Print and shaded views of the part. All mm, measured from the part's lowest x, y and z. A direction names the side the tool comes from. Coordinates: 2 decimals unless noted, no trailing zeros. Loops run counter-clockwise (first coordinate to the right, second up) from the corner with the lowest first, then second, coordinate; pieces in that order, holes last.
1) Saw through at C-C, the plane z = 6. Write the cut outline in (x, y), and give its area (3 significant figures).
2) Two-plate mould, pull along X, no slides. Class the marked faces 6, 7 and 8: +X half, -X half, draft (parallel to the pull), parting line (faces both ways), or undercut.
3) Saw through at D-D, the plane z = 10. Write the cut outline in (x, y), and give its area (3 significant figures).
4) Pin check, flat tips, straight feed: pin 1 Ø2 at (x, z) = (66, 2) entering from +Y; pin 2 Ø2.5 at (x, z) = (6, 6) entering from -Y; pin 3 Ø6 at (y, z) = (9, 5.5) entering from +X; pin 4 Ø6 at (y, z) = (9, 7) entering from -X. Stop position of each tip, or through.
5) Saw through at A-A, the plane y = 1.5. Write the cut outline in (x, z), and give its area (3 significant figures).
6) Which spindle directions (+Z, -Z, +X, -X, +Y, -Y) get a long thin tool onto all of the face, cutting with end or side? Do the marked faces 1, 2, 3, 4 and 5. Say none if no direction does.
7) Wall check: line 1 along Z through (x, y) = (6, 1.6); line 2 along X through (y, z) = (9.25, 7.75); line 3 along X through (y, z) = (10.75, 11). Give the ranges that are in metal, low to high.
8) Saw through at B-B, the plane x = 68. Write the cut outline in (y, z).
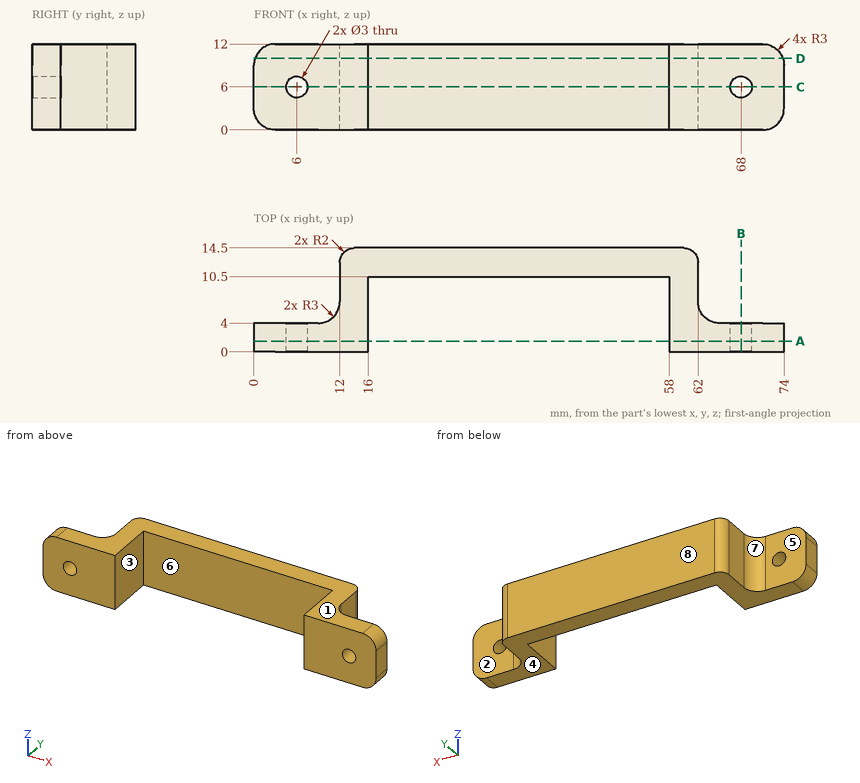
Data:
1. outline: (0, 0) - (4.5, 0) - (4.5, 4) - (0, 4) - close; (7.5, 0) - (16, 0) - (16, 10.5) - (58, 10.5) - (58, 0) - (66.5, 0) - (66.5, 4) - (65, 4) arc R3 cw to (62, 7) - (62, 12.5) arc R2 ccw to (60, 14.5) - (14, 14.5) arc R2 ccw to (12, 12.5) - (12, 7) arc R3 cw to (9, 4) - (7.5, 4) - close; (69.5, 0) - (74, 0) - (74, 4) - (69.5, 4) - close
1. area: 358 mm2
2. face 6: undercut
2. face 7: -X half
2. face 8: draft
3. outline: (0.17, 0) - (16, 0) - (16, 10.5) - (58, 10.5) - (58, 0) - (73.83, 0) - (73.83, 4) - (65, 4) arc R3 cw to (62, 7) - (62, 12.5) arc R2 ccw to (60, 14.5) - (14, 14.5) arc R2 ccw to (12, 12.5) - (12, 7) arc R3 cw to (9, 4) - (0.17, 4) - close
3. area: 381 mm2
4. pin 1: stops at y = 4
4. pin 2: passes through
4. pin 3: stops at x = 62.17
4. pin 4: stops at x = 11.83
5. outline: (0, 3) arc R3 ccw to (3, 0) - (16, 0) - (16, 12) - (3, 12) arc R3 ccw to (0, 9) - close; (58, 0) - (71, 0) arc R3 ccw to (74, 3) - (74, 9) arc R3 ccw to (71, 12) - (58, 12) - close; hole circle Ø3 at (6, 6); hole circle Ø3 at (68, 6)
5. area: 362 mm2
6. face 1: +Z, +X, -X, +Y, -Y
6. face 2: +Z, -Z, +X, +Y
6. face 3: +Z, -Z, -Y
6. face 4: -Z, +X, -X, +Y, -Y
6. face 5: +Z, -Z, -X, +Y
7. line 1: z = 0 to 4.5, 7.5 to 12
7. line 2: x = 12 to 16, 58 to 62
7. line 3: x = 12 to 62
8. outline: (0, 0) - (4, 0) - (4, 4.5) - (0, 4.5) - close; (0, 7.5) - (4, 7.5) - (4, 12) - (0, 12) - close
